Work out the finished part from the listing and answer in its coordinate system (mm). A direction names the side the tool comes from. Coordinates: 2 decimals unless noted, no trailing zeros. Order: outer loops, then holes, each group sorted by start corner. A loop starts at its lowest first (then second) coordinate and runs counter-clockwise, first axis right, second up. Notation, with made-up numbers: M 65,-38 L 92,-38 A11 ccw 92,-34 Z; hole C 50.25,25.25 d3. An arc over 180 degrees is marked long. Write item = value, one per line. Start each with the question number.
Q1. Find section A-A on y = 8.5. Give the vertices of the cut face in (x, z), and give its area (3 significant figures).
Q2. Find section B-B on z = 3.5. Give the number of separate pieces and of enclosed holes in the cut face, and give its area (3 significant figures).
Q3. Determine the mould class of faces 1 (the cylindrical face through (-1.04, 7.521, -2.546)), 2 (the cylindrical face through (-9.76, 1.92, -2.17)), 3 (the flat face through (-2, 0, 2)) for opening direction X: released by +X, released by -X, zero draft, split by the parting line, or undercut.
Q4. Find section C-C on y = 1.5. Give the vertices of the cut face in (x, z), and give its area (3 significant figures).
Q5. Each of these flat-tipped pins is pushed along its axis until it touches: P1, Ø3, axis at x = 0, z = 0, coming from the -Y side; P2, Ø2, axis at x = 1.5, y = 5, coming from the +Z side; P3, Ø1.5, axis at x = 0, y = 6.5, coming from the -Z side; P4, Ø1.8, axis at x = 6.6, z = 4.43, coming from the -Y side (3 decimals). Where does it stop, or does it pass through?
Q6. Straight lines are drawn through the part: line 1 along Z through (x, y) = (1.75, 2); line 2 along X through (y, z) = (1.7, 3.5); line 3 along Z through (x, y) = (-0.25, 1.5). For each, find the intervals that lie inside material, in ascending order.
Q7. A tool of negligible diameter and unlimited length cuts with its end or side. For faces 4 (the cylindrical face through (-2.44, 2.46, 0.54)), 5 (the cylindrical face through (1.064, 7.521, -2.536)), 6 (the flat face through (-2, 9, -2)), from which of +Z, -Z, +X, -X, +Y, -Y can it reach the whole face along a straight path? Write none if from no direction.
Q8. Find section D-D on y = 4. Give the vertices of the cut face in (x, z), and give its area (3 significant figures).
```python
from build123d import *

# Parameters (mm, degrees)
SKETCH1_R           = 10
BOSS_EXTRUDE1_DEPTH = 3
SKETCH2_R           = 4
BOSS_EXTRUDE2_DEPTH = 3
SKETCH3_R           = 2.5
CUT_EXTRUDE1_DEPTH  = 5
SKETCH4_R           = 1.5
CUT_EXTRUDE2_DEPTH  = 3
SKETCH5_R           = 0.925
CUT_EXTRUDE3_DEPTH  = 1
CHAMFER1_SIZE       = 0.5
CHAMFER1_SIZE2      = 0.866025404
SKETCH6_R           = 4
BOSS_EXTRUDE3_DEPTH = 3
SKETCH7_R           = 2.75
CUT_EXTRUDE4_DEPTH  = 3
BOSS_EXTRUDE6_DEPTH = 3


with BuildPart() as part:
    # Sketch1 → Boss-Extrude1 (new body)
    with BuildSketch(Plane(origin=(0, 0, 0), x_dir=(1, 0, 0), z_dir=(0, 1, 0))):
        with Locations(Location((0, 0, 0), (0, 0, 270))):
            Circle(SKETCH1_R)
    extrude(amount=BOSS_EXTRUDE1_DEPTH)

    # Sketch2 → Boss-Extrude2 (add)
    with BuildSketch(Plane(origin=(0, 3, 0), x_dir=(1, 0, 0), z_dir=(0, 1, 0))):
        with Locations(Location((0, 0, 0), (0, 0, 270))):
            Circle(SKETCH2_R)
    extrude(amount=BOSS_EXTRUDE2_DEPTH)

    # Sketch3 → Cut-Extrude1 (cut)
    with BuildSketch(Plane.XZ):
        with Locations(Location((0, 0, 0), (0, 0, 270))):
            Circle(SKETCH3_R)
    extrude(amount=-CUT_EXTRUDE1_DEPTH, mode=Mode.SUBTRACT)

    # Sketch4 → Cut-Extrude2 (cut)
    with BuildSketch(Plane.XZ):
        with Locations(Location((-7.141738564, 3.5, 0), (0, 0, 270))):
            Circle(SKETCH4_R)
        with Locations(Location((6.601958195, 4.434927024, 0), (0, 0, 270))):
            Circle(SKETCH4_R)
        with Locations(Location((0.539780369, -7.934927024, 0), (0, 0, 270))):
            Circle(SKETCH4_R)
    extrude(amount=-CUT_EXTRUDE2_DEPTH, mode=Mode.SUBTRACT)

    # Sketch5 → Cut-Extrude3 (cut)
    with BuildSketch(Plane(origin=(0, 6, 0), x_dir=(1, 0, 0), z_dir=(0, 1, 0))):
        with Locations(Location((0, 0, 0), (0, 0, 270))):
            Circle(SKETCH5_R)
    extrude(amount=-CUT_EXTRUDE3_DEPTH, mode=Mode.SUBTRACT)

    # Chamfer1
    chamfer1_edges = [part.edges().sort_by_distance(p)[0] for p in [
        (0, 0, -10),
    ]]
    chamfer1_side = [part.faces().sort_by_distance(p)[0] for p in [
        (0, 0, -9.717157288),
    ]]
    chamfer(chamfer1_edges, length=CHAMFER1_SIZE, length2=CHAMFER1_SIZE2, reference=chamfer1_side[0])

    # Sketch6 → Boss-Extrude3 (add)
    with BuildSketch(Plane(origin=(0, 6, 0), x_dir=(1, 0, 0), z_dir=(0, 1, 0))):
        with Locations(Location((0, 0, 0), (0, 0, 270))):
            Circle(SKETCH6_R)
    extrude(amount=BOSS_EXTRUDE3_DEPTH)

    # Sketch7 → Cut-Extrude4 (cut)
    with BuildSketch(Plane(origin=(0, 9, 0), x_dir=(1, 0, 0), z_dir=(0, 1, 0))):
        with Locations(Location((0, 0, 0), (0, 0, 270))):
            Circle(SKETCH7_R)
    extrude(amount=-CUT_EXTRUDE4_DEPTH, mode=Mode.SUBTRACT)

    # Sketch8 → Boss-Extrude6 (add)
    with BuildSketch(Plane(origin=(0, 6, 0), x_dir=(1, 0, 0), z_dir=(0, 1, 0))):
        Polygon((0, 2.5), (0.216506351, 2.875), (-0.216506351, 2.875), align=None)
        Polygon((1.767766953, 1.767766953), (2.186025105, 1.879838887), (1.879838887, 2.186025105), align=None)
        Polygon((2.5, 0), (2.875, -0.216506351), (2.875, 0.216506351), align=None)
        Polygon((1.767766953, -1.767766953), (1.879838887, -2.186025105), (2.186025105, -1.879838887), align=None)
        Polygon((0, -2.5), (-0.216506351, -2.875), (0.216506351, -2.875), align=None)
        Polygon((-1.767766953, -1.767766953), (-2.186025105, -1.879838887), (-1.879838887, -2.186025105), align=None)
        Polygon((-2.5, 0), (-2.875, 0.216506351), (-2.875, -0.216506351), align=None)
        Polygon((-1.767766953, 1.767766953), (-1.879838887, 2.186025105), (-2.186025105, 1.879838887), align=None)
    extrude(amount=BOSS_EXTRUDE6_DEPTH)


solid = part.part
```
Findings below:
q1.outline = C 0,0 d8; hole M -2.75,-0.14 A2.75 ccw -2.04,-1.84 L -1.77,-1.77 L -1.84,-2.04 A2.75 ccw -0.14,-2.75 L 0,-2.5 L 0.14,-2.75 A2.75 ccw 1.84,-2.04 L 1.77,-1.77 L 2.04,-1.84 A2.75 ccw 2.75,-0.14 L 2.5,0 L 2.75,0.14 A2.75 ccw 2.04,1.84 L 1.77,1.77 L 1.84,2.04 A2.75 ccw 0.14,2.75 L 0,2.5 L -0.14,2.75 A2.75 ccw -1.84,2.04 L -1.77,1.77 L -2.04,1.84 A2.75 ccw -2.75,0.14 L -2.5,0 Z
q1.area = 26.8 mm^2
q2.separate_pieces = 3
q2.enclosed_holes = 0
q2.area = 62.9 mm^2
q3.face_1 = undercut
q3.face_2 = split by the parting line
q3.face_3 = zero draft
q4.outline = C 0,0 d20; hole C -7.14,3.5 d3; hole C 0,0 d5; hole C 0.54,-7.93 d3; hole C 6.6,4.43 d3
q4.area = 273 mm^2
q5.P1 = 5
q5.P2 = 3.97
q5.P3 = -4
q5.P4 = through
q6.line_1 = -9.85 to -8.82, -7.05 to -1.79, 1.79 to 9.85
q6.line_2 = -9.37 to -8.64, -5.64 to 5.43, 7.77 to 9.37
q6.line_3 = -10 to -9.21, -6.66 to -2.49, 2.49 to 10
q7.face_4 = -Y
q7.face_5 = +Y
q7.face_6 = +Z, -Z, +X, -X, +Y
q8.outline = C 0,0 d8; hole C 0,0 d5
q8.area = 30.6 mm^2
